CAD build for the part. Positions are in the model's coordinates, mm. A direction names the side the tool comes from. Round coordinates to 2 decimals unless told otherwise and drop trailing zeros. Loops run counter-clockwise (first coordinate to the right, second up) from the corner with the lowest first, then second, coordinate; pieces in that order, holes last. Notation, with made-up numbers: M 21.25,-20 L 32.25,-20 A14 ccw 32.25,-4 Z; hole C 37.5,74.25 d3. An arc over 180 degrees is marked long. One line per item, written item: value. Start each with the question number.
from build123d import *

# Parameters (mm, degrees)
F0_W     = 24
F0_H     = 40.5
F1_DEPTH = 3
F2_R     = 1.5
F3_DEPTH = 25
F4_R     = 2.5
F5_W     = 4
F5_H     = 6
F6_DEPTH = 12.5
F7_W     = 16
F7_H     = 10
F8_DEPTH = 12.5
F9_SIZE  = 0.5


with BuildPart() as f1:
    # F0 (on Top) → F1 (new body, symmetric)
    with BuildSketch(Plane.XY):
        Rectangle(F0_W, F0_H)
    extrude(amount=F1_DEPTH, both=True)

    # F2 (on Right) → F3 (cut, symmetric)
    with BuildSketch(Plane.YZ):
        with Locations((-17.75, 0)):
            Circle(F2_R)
    extrude(amount=F3_DEPTH, both=True, mode=Mode.SUBTRACT)

    # F4
    f4_edges = [f1.edges().sort_by_distance(p)[0] for p in [
        (0, -20.25, 3),
        (0, -20.25, -3),
        (0, 20.25, 3),
        (0, 20.25, -3),
    ]]
    fillet(f4_edges, radius=F4_R)

    # F5 (on Top) → F6 (cut, symmetric)
    with BuildSketch(Plane.XY):
        with Locations((0, -17.25)):
            Rectangle(F5_W, F5_H)
        with Locations((-7, -17.25)):
            Rectangle(F5_W, F5_H)
        with Locations((7, -17.25)):
            Rectangle(F5_W, F5_H)
    extrude(amount=F6_DEPTH, both=True, mode=Mode.SUBTRACT)

    # F7 (on Top) → F8 (cut, symmetric)
    with BuildSketch(Plane.XY):
        with Locations((0, 7)):
            Rectangle(F7_W, F7_H)
    extrude(amount=F8_DEPTH, both=True, mode=Mode.SUBTRACT)

    # F9
    f9_edges = [f1.edges().sort_by_distance(p)[0] for p in [
        (12, 0, -3),
        (9, -19.517767, -2.267767),
        (5, -19.517767, -2.267767),
        (2, -19.517767, -2.267767),
        (-2, -19.517767, -2.267767),
        (-7, -14.25, -3),
        (-5, -19.517767, -2.267767),
        (-9, -19.517767, -2.267767),
        (-12, -19.517767, -2.267767),
        (0, -14.25, -3),
        (7, -14.25, -3),
    ]]
    chamfer(f9_edges, length=F9_SIZE)


solid = f1.part
(1) Probe L1, parallel to X at y = -18, z = -1.75; L2, parallel to Z at x = -10.55, y = -17.75; L3, parallel to Y at x = 0.5, z = 2. List the from-to ranges inside material, lowest first.
(2) Mould opens along X. For faces 1 (the conical face through (-11.86, 19.25, -2.03)), 2 (the cylindrical face through (-3.486, -19.537, 2.248)), 3 (the conical face through (4.86, -19.25, 2.03)) say: pulls with the +X half, pulls with the -X half, needs draft (parallel to the pull), parting line crosses it, or undercut.
(3) Slice it at A-A, the plane x = 3.5. List the corners of the cut face in (y, z), and give its area (3 significant figures).
(4) Which spindle directions (+Z, -Z, +X, -X, +Y, -Y) get a long thin tool onto all of the face, cutting with end or side? Do faces 4 (the conical face through (-2.135, -19.243, 2.026)), 5 (the flat face through (5, -16, 0)), 6 (the conical face through (2.135, -19.276, -1.993)), 7 (the flat face through (0, 20.25, 0)), 8 (the flat face through (0, 2, 0)). Say none if no direction does.
(5) Slice it at C-C, the plane z = 0. Count the separate pieces of the cut face and the enclosed holes in it, and give its area (3 significant figures).
(6) Slice it at B-B, the plane x = 8.5. List the corners of the cut face in (y, z).
(7) Flat gauge pins, fed straight in: P1, Ø1.5, axis at y = -17, z = -0.5, coming from the -X side; P2, Ø1.5, axis at x = -7.5, z = -0.5, coming from the -Y side; P3, Ø1.5, axis at x = -9.5, z = 1.5, coming from the -Y side. Where does each tip first touch, or does it go through?
Check result:
1. L1: x = -12 to -9, -5 to -2, 2 to 5, 9 to 12
1. L2: z = -3 to -1.5, 1.5 to 3
1. L3: y = -14.25 to 2, 12 to 19.75
2. face 1: pulls with the -X half
2. face 2: needs draft
2. face 3: undercut
3. outline: M -20.25,-0.5 A2.5 ccw -17.75,-3 L 2,-3 L 2,3 L -17.75,3 A2.5 ccw -20.25,0.5 Z; M 12,-3 L 17.75,-3 A2.5 ccw 20.25,-0.5 L 20.25,0.5 A2.5 ccw 17.75,3 L 12,3 Z; hole C -17.75,0 d3
3. area: 171 mm^2
4. face 4: +Z, -Y
4. face 5: +Z, -Z, -Y
4. face 6: -Z, -Y
4. face 7: +Z, -Z, +X, -X, +Y
4. face 8: +Z, -Z
5. separate pieces: 5
5. enclosed holes: 1
5. area: 703 mm^2
6. outline: M -14.25,-2.5 L -13.75,-3 L 17.75,-3 A2.5 ccw 20.25,-0.5 L 20.25,0.5 A2.5 ccw 17.75,3 L -14.25,3 Z
7. P1: stops at x = -12
7. P2: stops at y = -14.25
7. P3: stops at y = -20.24
